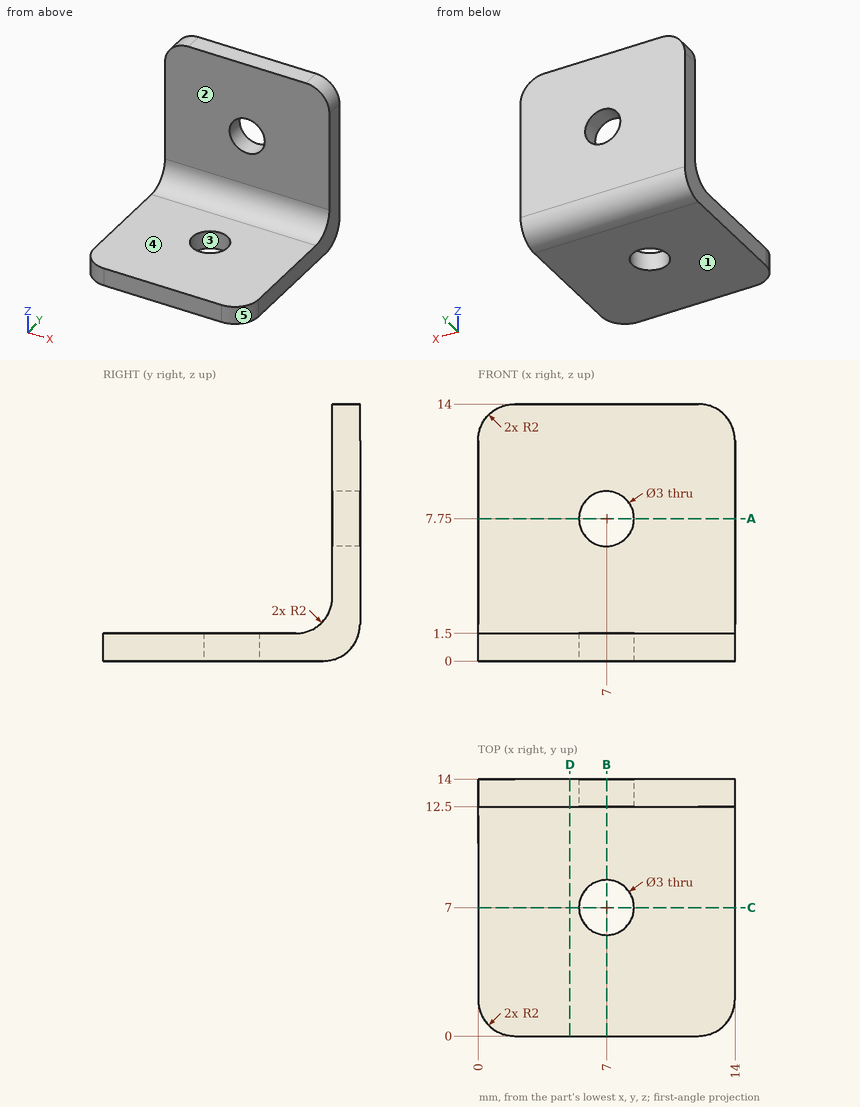
For this review, use the dimensioned drawing (mm, ordinates from the lowest corner) and the shaded views. A direction names the side the tool comes from. Coordinates: 2 decimals unless noted, no trailing zeros. Loops run counter-clockwise (first coordinate to the right, second up) from the corner with the lowest first, then second, coordinate; pieces in that order, holes last. Notation, with made-up numbers: (-30.5, 40) -> (-2.5, 40) arc R25 cw to (-2.5, 73) -> close; hole circle Ø10 at (-3, 60). An arc over 180 degrees is marked (long way). Use a Markdown table: item, result. Add a question column.
Item 1: We need section D-D, the plane x = 5. Write out the cut boundary in (y, z).
Item 2: We need section C-C, the plane y = 7. Write out the cut boundary in (x, z), and give its area (3 significant figures).
Item 3: Machinability: for the marked faces 4 and 5, which of the approach directions +Z, -Z, +X, -X, +Y, -Y give a long, thin tool a straight path to every point of the face, cutting with its end or side? Answer none if there is none.
Item 4: The part is to be moulded in two halves that separate along Y. For the marked faces 1, 2 and 3, say which applies: +Y half, -Y half, draft (parallel to the pull), parting line (faces both ways), or undercut.
Item 5: Wall thickness on L1, parallel to Z at x = 5.75, y = 3.25; L2, parallel to Y at x = 8.75, z = 7.5; L3, parallel to Y at x = 7, z = 0.4: over which ranges is each line inside the solid? List them lowest first. Write a range as from..to.
Item 6: Clearance check with flat-ended pins moving along their axes: P1, Ø2, axis at x = 8, z = 10, coming from the -Y side; P2, Ø8, axis at x = 6, y = 10, coming from the +Z side; P3, Ø2.5, axis at x = 7, y = 7, coming from the +Z side. State where each tip first meets the part, or that it passes through.
Item 7: We need section B-B, the plane x = 7. Write out the cut boundary in (y, z).
Item 8: We need section A-A, the plane z = 7.75. Write out the cut boundary in (x, y).
Numbers:
| question | item | result |
|---|---|---|
| 1 | outline | (0, 0) -> (12, 0) arc R2 ccw to (14, 2) -> (14, 14) -> (12.5, 14) -> (12.5, 3.5) arc R2 cw to (10.5, 1.5) -> (0, 1.5) -> close |
| 2 | outline | (0, 0) -> (5.5, 0) -> (5.5, 1.5) -> (0, 1.5) -> close; (8.5, 0) -> (14, 0) -> (14, 1.5) -> (8.5, 1.5) -> close |
| 2 | area | 16.5 mm^2 |
| 3 | face 4 | +Z, +X, -X, -Y |
| 3 | face 5 | +Z, -Z, +X, -Y |
| 4 | face 1 | draft |
| 4 | face 2 | -Y half |
| 4 | face 3 | undercut |
| 5 | L1 | z = 0..1.5 |
| 5 | L2 | y = 12.5..14 |
| 5 | L3 | y = 0..5.5, 8.5..13.2 |
| 6 | P1 | stops at y = 12.5 |
| 6 | P2 | stops at z = 14 |
| 6 | P3 | passes through |
| 7 | outline | (0, 0) -> (5.5, 0) -> (5.5, 1.5) -> (0, 1.5) -> close; (8.5, 0) -> (12, 0) arc R2 ccw to (14, 2) -> (14, 6.25) -> (12.5, 6.25) -> (12.5, 3.5) arc R2 cw to (10.5, 1.5) -> (8.5, 1.5) -> close; (12.5, 9.25) -> (14, 9.25) -> (14, 14) -> (12.5, 14) -> close |
| 8 | outline | (0, 12.5) -> (5.5, 12.5) -> (5.5, 14) -> (0, 14) -> close; (8.5, 12.5) -> (14, 12.5) -> (14, 14) -> (8.5, 14) -> close |
